The listing builds one solid part. Answer for the finished solid, in the listing's coordinates (mm). A direction names the side the tool comes from. Give positions to 0.01 mm unless a question says otherwise; leave off trailing zeros. Loops run counter-clockwise (first coordinate to the right, second up) from the corner with the lowest first, then second, coordinate; pieces in that order, holes last. Notation, with made-up numbers: (40.25, -30.75) - (57.25, -30.75) arc R9 ccw to (57.25, -13.75) - close; hole circle Ø5 at (6.25, 31). An arc over 180 degrees is marked (long way). Answer in a Markdown table with one row per item. Add a question column.
Autodesk Inventor part; units mm, degrees
ref_plane "YZ Plane" through (0, 0, 0) normal (1, 0, 0) x (0, 1, 0)
ref_plane "XZ Plane" through (0, 0, 0) normal (0, 1, 0) x (-1, 0, 0)
ref_plane "XY Plane" through (0, 0, 0) normal (0, 0, 1) x (1, 0, 0)
sketch "Sketch1" plane through (0, 0, 0) normal (0, 1, 0) x (-1, 0, 0)
  line L0 (0, 0) -> (45, 0)
  line L1 (45, 0) -> (45, -6)
  line L2 (45, -6) -> (0, -6)
  line L3 (0, -6) -> (0, 0)
  dimension "d0" = 45
  dimension "d1" = 6
extrude "Extrusion1" add sketch "Sketch1" along normal blind 42
sketch "Sketch3" plane through (0, 0, 0) normal (0, -1, 0) x (1, 0, 0)
  line L0 (-12.5, 0) -> (-32.5, 0)
  line L1 (-22.5, 0) -> (-22.5, -3)
  line L2 (-22.5, -3) -> (-12.5, -3)
  line L3 (-22.5, -3) -> (-32.5, -3)
  point P0 (0, 0)
  dimension "d9" = 3
  dimension "d10" = 10
  dimension "d11" = 10
hole "Hole1" at (-12.5, 0, -3) at (-32.5, 0, -3) direction (0, 1, 0) diameter 4.5 depth 11 tip angle 118
sketch "Sketch4" plane through (-45, 0, 0) normal (0, 0, 1) x (1, 0, 0)
  line L0 (45, 0) -> (0, 0)
  line L1 (22.5, 0) -> (22.5, 22)
  circle A0 centre (22.5, 22) radius 16.5
  dimension "d19" = 22
  dimension "d20" = 33
extrude "Extrusion3" cut sketch "Sketch4" against normal through all
properties part number "Motor_Mount_Backplate"
(1) Given pin 1 Ø3.5 at (x, z) = (-12.5, -3) entering from -Y; pin 2 Ø5 at (x, y) = (-26, 33.5) entering from +Z, each flat-ended and moving along its own axis, determine where each tip first touches the part or whether it passes through.
(2) A cutting plane is placed at A-A on y = 22. Determine the outline of the cut face in (x, z).
(3) A cutting plane is placed at C-C on x = -12.5. Determine the outline of the cut face in (y, z).
(4) The mould has two halves that part along X. Classify faces 3 (the face through (0, 21, -3)), 4 (the face through (-45, 21, -3)), 5 (the face through (-7.26, 15.68, -2.96)): pulls with the +X half, pulls with the -X half, needs draft (parallel to the pull), parting line crosses it, or undercut.
(5) A cutting plane is placed at D-D on x = -23. Determine the outline of the cut face in (y, z).
(6) Find the intervals of material crossed by line 1 along X through (y, z) = (4.5, -3); line 2 along Y through (x, z) = (-22.5, -1.75); line 3 along Z through (x, y) = (-12.5, 8), in increasing order. Write a range as [from, to].
(7) A tool of negligible diameter and unlimited length cuts with its end or side. For faces 1 (the face through (-10.504, 4.334, -4.038)), 2 (the face through (-22, 0, -3)), from which of +Z, -Z, +X, -X, +Y, -Y can it reach the whole face along a straight path? Write none if from no direction.
(8) A cutting plane is placed at B-B on z = -3. Determine the outline of the cut face in (x, y).
Evaluation:
| question | item | result |
|---|---|---|
| 1 | pin 1 | stops at y = 33.58 |
| 1 | pin 2 | passes through |
| 2 | outline | (-45, -6) - (-39, -6) - (-39, 0) - (-45, 0) - close; (-6, -6) - (0, -6) - (0, 0) - (-6, 0) - close |
| 3 | outline | (0, -6) - (8.88, -6) - (8.88, -5.25) - (0, -5.25) - close; (0, -0.75) - (8.88, -0.75) - (8.88, 0) - (0, 0) - close; (35.12, -6) - (42, -6) - (42, 0) - (35.12, 0) - close |
| 4 | face 3 | pulls with the +X half |
| 4 | face 4 | pulls with the -X half |
| 4 | face 5 | undercut |
| 5 | outline | (0, -6) - (5.51, -6) - (5.51, 0) - (0, 0) - close; (38.49, -6) - (42, -6) - (42, 0) - (38.49, 0) - close |
| 6 | line 1 | x = [-45, -34.75], [-30.25, -14.75], [-10.25, 0] |
| 6 | line 2 | y = [0, 5.5], [38.5, 42] |
| 6 | line 3 | z = [-6, -5.25], [-0.75, 0] |
| 7 | face 1 | -Y |
| 7 | face 2 | +Z, -Z, +X, -X, -Y |
| 8 | outline | (-45, 0) - (-34.75, 0) - (-34.75, 10.95) arc R16.5 cw (long way) to (-10.25, 10.95) - (-10.25, 0) - (0, 0) - (0, 42) - (-45, 42) - close; (-30.25, 0) - (-14.75, 0) - (-14.75, 7.43) arc R16.5 cw to (-30.25, 7.43) - close |
